Input: part model. Units: mm. Frame: model coordinates. Round coordinates to 2 decimals unless told otherwise and drop trailing zeros. Loops run counter-clockwise (first coordinate to the right, second up) from the corner with the lowest first, then second, coordinate; pieces in that order, holes last. Notation, with made-up numbers: M 25,55.5 L 59,55.5 A14 cw 59,77.5 Z; hole C 61,12.5 d7. An arc over 180 degrees is marked long. Return JSON: item names as keys, results as strings. Group by question number.
1) Material intervals for line 1 (X direction, y = 1.85, z = 2); line 2 (Z direction, x = 39, y = 1.8); line 3 (Z direction, x = 103, y = 2.1), sorted ascending. Write a range as from..to.
2) Section A-A (x = -46). Output: boundary loops of the cut face in (y, z), plus the area to 3 significant figures.
3) Contact query for a flat-ended pin moving along its axis: P1, Ø1.5, axis at x = 77.5, z = -18, coming from the +Y side. Output: stop coordinate, or through.
4) Section B-B (y = 2.95). Count the separate pieces of the cut face and the enclosed holes in it, plus the area to 3 significant figures.
from build123d import *

# Parameters (mm, degrees)
SKETCH_1_W          = 250
SKETCH_1_H          = 230
EXTRUDE_1_DEPTH     = 4
SKETCH_5_R          = 1.55
CUT_EXTRUDE_4_DEPTH = 3
SKETCH_7_R          = 1.5
CUT_EXTRUDE_5_DEPTH = 170.899970571
SKETCH_8_W          = 250
SKETCH_8_H          = 8
CUT_EXTRUDE_6_DEPTH = 10
SKETCH_9_W          = 250
SKETCH_9_H          = 8
EXTRUDE_2_DEPTH     = 4
CHAMFER_1_SIZE      = 5
FILLET_1_R          = 1


with BuildPart() as part:
    # 草图1 → 凸台-拉伸1 (new body)
    with BuildSketch(Plane(origin=(0, 0, 0), x_dir=(1, 0, 0), z_dir=(0, 1, 0))):
        Rectangle(SKETCH_1_W, SKETCH_1_H)
    extrude(amount=EXTRUDE_1_DEPTH)

    # 草图5 → 切除-拉伸4 (cut)
    with BuildSketch(Plane(origin=(0, 4, 0), x_dir=(1, 0, 0), z_dir=(0, 1, 0))):
        with Locations(Location((77.5, -2, 0), (0, 0, 270))):
            Circle(SKETCH_5_R)
        with Locations(Location((77.5, 18, 0), (0, 0, 270))):
            Circle(SKETCH_5_R)
        with Locations(Location((77.5, -22, 0), (0, 0, 90))):
            Circle(SKETCH_5_R)
        with Locations(Location((77.5, -42, 0), (0, 0, 90))):
            Circle(SKETCH_5_R)
        with Locations(Location((-77.5, -42, 0), (0, 0, 270))):
            Circle(SKETCH_5_R)
        with Locations(Location((-77.5, -22, 0), (0, 0, 270))):
            Circle(SKETCH_5_R)
        with Locations(Location((-77.5, 18, 0), (0, 0, 90))):
            Circle(SKETCH_5_R)
        with Locations(Location((-77.5, -2, 0), (0, 0, 90))):
            Circle(SKETCH_5_R)
    extrude(amount=-CUT_EXTRUDE_4_DEPTH, mode=Mode.SUBTRACT)

    # 草图7 → 切除-拉伸5 (cut, through all)
    with BuildSketch(Plane(origin=(0, 4, 0), x_dir=(1, 0, 0), z_dir=(0, 1, 0))):
        with Locations(Location((-117.000000001, 94.78695798, 0), (0, 0, 270))):
            Circle(SKETCH_7_R)
        with Locations(Location((-117.000000001, 70.78695798, 0), (0, 0, 270))):
            Circle(SKETCH_7_R)
        with Locations(Location((-103.000000001, 70.78695798, 0), (0, 0, 270))):
            Circle(SKETCH_7_R)
        with Locations(Location((-103.000000001, 94.78695798, 0), (0, 0, 270))):
            Circle(SKETCH_7_R)
        with Locations(Location((-7, 94.786957979, 0), (0, 0, 270))):
            Circle(SKETCH_7_R)
        with Locations(Location((7, 94.786957979, 0), (0, 0, 270))):
            Circle(SKETCH_7_R)
        with Locations(Location((7, 70.786957979, 0), (0, 0, 270))):
            Circle(SKETCH_7_R)
        with Locations(Location((-7, 70.786957979, 0), (0, 0, 270))):
            Circle(SKETCH_7_R)
        with Locations(Location((116.999999999, 94.78695798, 0), (0, 0, 270))):
            Circle(SKETCH_7_R)
        with Locations(Location((116.999999999, 70.78695798, 0), (0, 0, 270))):
            Circle(SKETCH_7_R)
        with Locations(Location((102.999999999, 70.78695798, 0), (0, 0, 270))):
            Circle(SKETCH_7_R)
        with Locations(Location((102.999999999, 94.78695798, 0), (0, 0, 270))):
            Circle(SKETCH_7_R)
        with Locations(Location((103, -109.213042021, 0), (0, 0, 270))):
            Circle(SKETCH_7_R)
        with Locations(Location((117, -109.213042021, 0), (0, 0, 270))):
            Circle(SKETCH_7_R)
        with Locations(Location((117, -85.213042021, 0), (0, 0, 270))):
            Circle(SKETCH_7_R)
        with Locations(Location((103, -85.213042021, 0), (0, 0, 270))):
            Circle(SKETCH_7_R)
        with Locations(Location((7, -85.213042021, 0), (0, 0, 270))):
            Circle(SKETCH_7_R)
        with Locations(Location((7, -109.213042021, 0), (0, 0, 270))):
            Circle(SKETCH_7_R)
        with Locations(Location((-7, -85.213042021, 0), (0, 0, 270))):
            Circle(SKETCH_7_R)
        with Locations(Location((-7, -109.213042021, 0), (0, 0, 270))):
            Circle(SKETCH_7_R)
        with Locations(Location((-117, -85.213042021, 0), (0, 0, 270))):
            Circle(SKETCH_7_R)
        with Locations(Location((-103, -85.213042021, 0), (0, 0, 270))):
            Circle(SKETCH_7_R)
        with Locations(Location((-103, -109.213042021, 0), (0, 0, 270))):
            Circle(SKETCH_7_R)
        with Locations(Location((-117, -109.213042021, 0), (0, 0, 270))):
            Circle(SKETCH_7_R)
    extrude(amount=-CUT_EXTRUDE_5_DEPTH, mode=Mode.SUBTRACT)

    # 草图8 → 切除-拉伸6 (cut)
    with BuildSketch(Plane(origin=(0, 4, 0), x_dir=(1, 0, 0), z_dir=(0, 1, 0))):
        with BuildLine():
            Line((-73, 97), (-38, 97))
            ThreePointArc((-38, 97), (-34.5, 93.5), (-38, 90))
            Line((-38, 90), (-73, 90))
            ThreePointArc((-73, 90), (-76.5, 93.5), (-73, 97))
        make_face()
        with BuildLine():
            Line((-73, 79), (-38, 79))
            ThreePointArc((-38, 79), (-34.5, 75.5), (-38, 72))
            Line((-38, 72), (-73, 72))
            ThreePointArc((-73, 72), (-76.5, 75.5), (-73, 79))
        make_face()
        with BuildLine():
            Line((73, 97), (38, 97))
            ThreePointArc((38, 97), (34.5, 93.5), (38, 90))
            Line((38, 90), (73, 90))
            ThreePointArc((73, 90), (76.5, 93.5), (73, 97))
        make_face()
        with BuildLine():
            Line((73, 79), (38, 79))
            ThreePointArc((38, 79), (34.5, 75.5), (38, 72))
            Line((38, 72), (73, 72))
            ThreePointArc((73, 72), (76.5, 75.5), (73, 79))
        make_face()
        with BuildLine():
            Line((-73, -97), (-38, -97))
            ThreePointArc((-38, -97), (-34.5, -93.5), (-38, -90))
            Line((-38, -90), (-73, -90))
            ThreePointArc((-73, -90), (-76.5, -93.5), (-73, -97))
        make_face()
        with BuildLine():
            Line((-73, -79), (-38, -79))
            ThreePointArc((-38, -79), (-34.5, -75.5), (-38, -72))
            Line((-38, -72), (-73, -72))
            ThreePointArc((-73, -72), (-76.5, -75.5), (-73, -79))
        make_face()
        with BuildLine():
            Line((73, -97), (38, -97))
            ThreePointArc((38, -97), (34.5, -93.5), (38, -90))
            Line((38, -90), (73, -90))
            ThreePointArc((73, -90), (76.5, -93.5), (73, -97))
        make_face()
        with BuildLine():
            Line((73, -79), (38, -79))
            ThreePointArc((38, -79), (34.5, -75.5), (38, -72))
            Line((38, -72), (73, -72))
            ThreePointArc((73, -72), (76.5, -75.5), (73, -79))
        make_face()
        with Locations((0, 111)):
            Rectangle(SKETCH_8_W, SKETCH_8_H)
    extrude(amount=-CUT_EXTRUDE_6_DEPTH, mode=Mode.SUBTRACT)

    # 草图9 → 凸台-拉伸2 (add)
    with BuildSketch(Plane(origin=(0, 4, 0), x_dir=(1, 0, 0), z_dir=(0, 1, 0))):
        with Locations((0, -119)):
            Rectangle(SKETCH_9_W, SKETCH_9_H)
    extrude(amount=-EXTRUDE_2_DEPTH)

    # 倒角1
    chamfer_1_edges = [part.edges().sort_by_distance(p)[0] for p in [
        (-125, 2, -107),
        (125, 2, -107),
        (-125, 2, 123),
        (125, 2, 123),
    ]]
    chamfer(chamfer_1_edges, length=CHAMFER_1_SIZE)

    # 圆角1
    fillet_1_edges = [part.edges().sort_by_distance(p)[0] for p in [
        (-125, 2, -102),
        (-125, 2, 118),
        (120, 2, 123),
        (-120, 2, 123),
        (125, 2, 118),
        (125, 2, -102),
        (-120, 2, -107),
        (120, 2, -107),
    ]]
    fillet(fillet_1_edges, radius=FILLET_1_R)


solid = part.part
Returned:
{
 "1": {"line 1": "x = -125..-79.05, -75.95..75.95, 79.05..125", "line 2": "z = -107..-97, -90..-79, -72..72, 79..90, 97..123", "line 3": "z = -107..-96.29, -93.29..-72.29, -69.29..83.71, 86.71..107.71, 110.71..123"},
 "2": {"outline": "M 0,-107 L 4,-107 L 4,-97 L 0,-97 Z; M 0,-90 L 4,-90 L 4,-79 L 0,-79 Z; M 0,-72 L 4,-72 L 4,72 L 0,72 Z; M 0,79 L 4,79 L 4,90 L 0,90 Z; M 0,97 L 4,97 L 4,123 L 0,123 Z", "area": "808 mm^2"},
 "3": {"P1": "stops at y = 1"},
 "4": {"separate pieces": "1", "enclosed holes": "40", "area": "55,000 mm^2"}
}
